Read the model definition and answer for the solid it produces. Units are mm, in the model's axes. A direction names the side the tool comes from. Give positions to 0.01 mm unless a question says otherwise; leave off trailing zeros. Loops run counter-clockwise (first coordinate to the right, second up) from the corner with the lowest first, then second, coordinate; pieces in that order, holes last. Notation, with made-up numbers: (36, -14.75) -> (82, -14.75) arc R34 cw to (82, 21.25) -> close; hole circle Ø9 at (37.5, 20). An arc over 180 degrees is marked (long way). Return JSON: item names as keys, results as strings. Group by question number.
from build123d import *

# Parameters (mm, degrees)
ESBO_O1_W                = 100
ESBO_O1_H                = 180
ESBO_O1_R                = 24
ESBO_O1_W_2              = 80
ESBO_O1_H_2              = 50.3
RESSALTO_EXTRUS_O1_DEPTH = 20
CORTE_EXTRUS_O1_DEPTH    = 227.2
FILETE1_R                = 50
FILETE2_R                = 8
FILETE3_R                = 1.5
CASCA1_T                 = -2.5
CORTE_EXTRUS_O2_START    = 108.4
ESBO_O3_R                = 26.5
CORTE_EXTRUS_O2_DEPTH    = 105.4
ESBO_O4_W                = 85
ESBO_O4_H                = 55.3
CORTE_EXTRUS_O3_DEPTH    = 17.5


with BuildPart() as part:
    # Esboço1 → Ressalto-extrusão1 (new body)
    # profile 1 of 13: a face of its own
    with BuildSketch(Plane.XY):
        with Locations((50, 90)):
            Rectangle(ESBO_O1_W, ESBO_O1_H)
        with Locations((50, 59.7)):
            Circle(ESBO_O1_R, mode=Mode.SUBTRACT)
        with Locations((50, 134.85)):
            Rectangle(ESBO_O1_W_2, ESBO_O1_H_2, mode=Mode.SUBTRACT)
    # profile 2 of 13: a face of its own
    with BuildSketch(Plane.XY):
        with BuildLine():
            ThreePointArc((58.75, 74.855444566), (50, 77.2), (41.25, 74.855444566))
            Line((41.25, 74.855444566), (46.25, 66.195190528))
            ThreePointArc((46.25, 66.195190528), (50, 67.2), (53.75, 66.195190528))
            Line((53.75, 66.195190528), (58.75, 74.855444566))
        make_face()
    # profile 3 of 13: a face of its own
    with BuildSketch(Plane.XY):
        with BuildLine():
            Line((46.25, 66.195190528), (41.25, 74.855444566))
            ThreePointArc((41.25, 74.855444566), (37.625631329, 72.074368671), (34.844555434, 68.45))
            Line((34.844555434, 68.45), (43.504809472, 63.45))
            ThreePointArc((43.504809472, 63.45), (44.696699141, 65.003300859), (46.25, 66.195190528))
        make_face()
    # profile 4 of 13: a face of its own
    with BuildSketch(Plane.XY):
        with BuildLine():
            Line((43.504809472, 63.45), (34.844555434, 68.45))
            ThreePointArc((34.844555434, 68.45), (32.5, 59.7), (34.844555434, 50.95))
            Line((34.844555434, 50.95), (43.504809472, 55.95))
            ThreePointArc((43.504809472, 55.95), (42.5, 59.7), (43.504809472, 63.45))
        make_face()
    # profile 5 of 13: a face of its own
    with BuildSketch(Plane.XY):
        with BuildLine():
            Line((43.504809472, 55.95), (34.844555434, 50.95))
            ThreePointArc((34.844555434, 50.95), (37.625631329, 47.325631329), (41.25, 44.544555434))
            Line((41.25, 44.544555434), (46.25, 53.204809472))
            ThreePointArc((46.25, 53.204809472), (44.696699141, 54.396699141), (43.504809472, 55.95))
        make_face()
    # profile 6 of 13: a face of its own
    with BuildSketch(Plane.XY):
        with BuildLine():
            Line((58.75, 44.544555434), (53.75, 53.204809472))
            ThreePointArc((53.75, 53.204809472), (50, 52.2), (46.25, 53.204809472))
            Line((46.25, 53.204809472), (41.25, 44.544555434))
            ThreePointArc((41.25, 44.544555434), (50, 42.2), (58.75, 44.544555434))
        make_face()
    # profile 7 of 13: a face of its own
    with BuildSketch(Plane.XY):
        with BuildLine():
            ThreePointArc((67.5, 59.7), (66.90370196, 64.229333289), (65.155444566, 68.45))
            Line((65.155444566, 68.45), (56.495190528, 63.45))
            ThreePointArc((56.495190528, 63.45), (57.244443697, 61.641142838), (57.5, 59.7))
            ThreePointArc((57.5, 59.7), (57.244443697, 57.758857162), (56.495190528, 55.95))
            Line((56.495190528, 55.95), (65.155444566, 50.95))
            ThreePointArc((65.155444566, 50.95), (66.90370196, 55.170666711), (67.5, 59.7))
        make_face()
    # profile 8 of 13: a face of its own
    with BuildSketch(Plane.XY):
        with BuildLine():
            ThreePointArc((56.495190528, 55.95), (55.303300859, 54.396699141), (53.75, 53.204809472))
            Line((53.75, 53.204809472), (58.75, 44.544555434))
            ThreePointArc((58.75, 44.544555434), (62.374368671, 47.325631329), (65.155444566, 50.95))
            Line((65.155444566, 50.95), (56.495190528, 55.95))
        make_face()
    # profile 9 of 13: a face of its own
    with BuildSketch(Plane.XY):
        with BuildLine():
            ThreePointArc((65.155444566, 68.45), (62.374368671, 72.074368671), (58.75, 74.855444566))
            Line((58.75, 74.855444566), (53.75, 66.195190528))
            ThreePointArc((53.75, 66.195190528), (55.303300859, 65.003300859), (56.495190528, 63.45))
            Line((56.495190528, 63.45), (65.155444566, 68.45))
        make_face()
    # profile 10 of 13: a face of its own
    with BuildSketch(Plane.XY):
        with BuildLine():
            Line((41.25, 74.855444566), (38, 80.484609691))
            ThreePointArc((38, 80.484609691), (33.029437252, 76.670562748), (29.215390309, 71.7))
            Line((29.215390309, 71.7), (34.844555434, 68.45))
            ThreePointArc((34.844555434, 68.45), (37.625631329, 72.074368671), (41.25, 74.855444566))
        make_face()
    # profile 11 of 13: a face of its own
    with BuildSketch(Plane.XY):
        with BuildLine():
            Line((34.844555434, 50.95), (29.215390309, 47.7))
            ThreePointArc((29.215390309, 47.7), (33.029437252, 42.729437252), (38, 38.915390309))
            Line((38, 38.915390309), (41.25, 44.544555434))
            ThreePointArc((41.25, 44.544555434), (37.625631329, 47.325631329), (34.844555434, 50.95))
        make_face()
    # profile 12 of 13: a face of its own
    with BuildSketch(Plane.XY):
        with BuildLine():
            ThreePointArc((62, 38.915390309), (66.970562748, 42.729437252), (70.784609691, 47.7))
            Line((70.784609691, 47.7), (65.155444566, 50.95))
            ThreePointArc((65.155444566, 50.95), (62.374368671, 47.325631329), (58.75, 44.544555434))
            Line((58.75, 44.544555434), (62, 38.915390309))
        make_face()
    # profile 13 of 13: a face of its own
    with BuildSketch(Plane.XY):
        with BuildLine():
            ThreePointArc((70.784609691, 71.7), (66.970562748, 76.670562748), (62, 80.484609691))
            Line((62, 80.484609691), (58.75, 74.855444566))
            ThreePointArc((58.75, 74.855444566), (62.374368671, 72.074368671), (65.155444566, 68.45))
            Line((65.155444566, 68.45), (70.784609691, 71.7))
        make_face()
    extrude(amount=RESSALTO_EXTRUS_O1_DEPTH)

    # Esboço2 → Corte-extrusão1 (cut)
    with BuildSketch(Plane.XY.offset(20)):
        Polygon((10, 45.85), (0, 91.7), (0, 0), (10, 0), align=None)
        Polygon((90, 45.85), (90, 0), (100, 0), (100, 91.7), align=None)
    extrude(amount=-CORTE_EXTRUS_O1_DEPTH, mode=Mode.SUBTRACT)

    # Filete1
    filete1_edges = [part.edges().sort_by_distance(p)[0] for p in [
        (90, 45.85, 10),
        (0, 91.7, 10),
        (10, 45.85, 10),
        (100, 91.7, 10),
    ]]
    fillet(filete1_edges, radius=FILETE1_R)

    # Filete2
    filete2_edges = [part.edges().sort_by_distance(p)[0] for p in [
        (90, 0, 10),
        (0, 180, 10),
        (100, 180, 10),
        (10, 0, 10),
    ]]
    fillet(filete2_edges, radius=FILETE2_R)

    # Filete3
    filete3_edges = [part.edges().sort_by_distance(p)[0] for p in [
        (58.75, 74.855444566, 10),
        (62, 80.484609691, 10),
        (38, 80.484609691, 10),
        (41.25, 74.855444566, 10),
        (34.844555434, 68.45, 10),
        (29.215390309, 71.7, 10),
        (29.215390309, 47.7, 10),
        (34.844555434, 50.95, 10),
        (70.784609691, 47.7, 10),
        (70.784609691, 71.7, 10),
        (65.155444566, 68.45, 10),
        (65.155444566, 50.95, 10),
        (41.25, 44.544555434, 10),
        (38, 38.915390309, 10),
        (62, 38.915390309, 10),
        (58.75, 44.544555434, 10),
    ]]
    fillet(filete3_edges, radius=FILETE3_R)

    # Casca1
    casca1_openings = [part.faces().sort_by_distance(p)[0] for p in [
        (50, 40.944516246, 0),
    ]]
    offset(amount=CASCA1_T, openings=casca1_openings, kind=Kind.INTERSECTION)

    # Esboço3 → Corte-extrusão2 (cut)
    with BuildSketch(Plane(origin=(0, 0, 17.5), x_dir=(-1, 0, 0), z_dir=(0, 0, -1)).offset(CORTE_EXTRUS_O2_START)):
        with Locations((-50, 59.7)):
            Circle(ESBO_O3_R)
    extrude(amount=-CORTE_EXTRUS_O2_DEPTH, mode=Mode.SUBTRACT)

    # Esboço4 → Corte-extrusão3 (cut)
    with BuildSketch(Plane(origin=(0, 0, 0), x_dir=(-1, 0, 0), z_dir=(0, 0, -1))):
        with Locations((-50, 134.85)):
            Rectangle(ESBO_O4_W, ESBO_O4_H)
    extrude(amount=-CORTE_EXTRUS_O3_DEPTH, mode=Mode.SUBTRACT)


solid = part.part
1. Determine the mould class of faces 4 (the cylindrical face through (2.766, 92.07, 8.628)), 5 (the flat face through (98, 117, 0)), 6 (the flat face through (10, 24, 10)) for opening direction X: pulls with the +X half, pulls with the -X half, needs draft (parallel to the pull), parting line crosses it, or undercut.
2. Straight lines are drawn through the part: line 1 (X direction, y = 18, z = 12.25); line 2 (X direction, y = 155.5, z = 8.75); line 3 (Y direction, x = 61.5, z = 4.5). For each, find the intervals that lie inside material, in ascending order. Write a range as from..to.
3. Flat-ended cylindrical pins translate along their axes: pin 1 Ø10.5 at (x, y) = (72.5, 63.5) entering from -Z; pin 2 Ø8 at (x, y) = (87.5, 123) entering from -Z; pin 3 Ø5 at (y, z) = (21.5, 8.5) entering from +X. Find the tip coordinate at first contact, or state that the pin passes through.
4. Which of the six approach directions +Z, -Z, +X, -X, +Y, -Y give full straight-line access (tool end or side, diameter ignored) to faces 1 (the cylindrical face through (49.9, 42.2, 17.2)), 2 (the cylindrical face through (87.594, 2.281, 9.86)), 3 (the cylindrical face through (4.07, 175.85, 8.87))?
5. Section A-A on y = 12 is taken. Determine the outline of the cut face in (x, z), then the cut area to 4 significant figures.
6. Section C-C on y = 122 is taken. Determine the outline of the cut face in (x, z), then the cut area to 4 significant figures.
Completed:
{
 "1": {"face 4": "undercut", "face 5": "needs draft", "face 6": "pulls with the -X half"},
 "2": {"line 1": "x = 10..12.5, 87.5..90", "line 2": "x = 0..2.5, 97.5..100", "line 3": "y = 0..2.5, 177.5..180"},
 "3": {"pin 1": "stops at z = 14.5", "pin 2": "stops at z = 17.5", "pin 3": "stops at x = 90"},
 "4": {"face 1": "+Z, -Z", "face 2": "+Z, -Z, +X, -Y", "face 3": "-Z"},
 "5": {"outline": "(10, 0) -> (12.5, 0) -> (12.5, 17.5) -> (87.5, 17.5) -> (87.5, 0) -> (90, 0) -> (90, 20) -> (10, 20) -> close", "area": "287.5 mm²"},
 "6": {"outline": "(0, 0) -> (2.5, 0) -> (2.5, 17.5) -> (10, 17.5) -> (10, 20) -> (0, 20) -> close; (90, 17.5) -> (97.5, 17.5) -> (97.5, 0) -> (100, 0) -> (100, 20) -> (90, 20) -> close", "area": "137.5 mm²"}
}
